The listing builds one solid part. Answer for the finished solid, in the listing's coordinates (mm). A direction names the side the tool comes from. Round coordinates to 2 decimals unless told otherwise and drop trailing zeros. Order: outer loops, then holes, each group sorted by start corner. A loop starts at its lowest first (then second) coordinate and runs counter-clockwise, first axis right, second up. Notation, with made-up numbers: M 28.5,-16 L 36.5,-16 A20 cw 36.5,-3 Z; hole C 46.25,57.5 d4. An arc over 180 degrees is marked long. Put each result on its own line as item: value. Start each with the question number.
1. Each of these flat-tipped pins is pushed along its axis until it touches: pin 1 Ø4 at (x, z) = (1.5, 3) entering from +Y; pin 2 Ø2 at (x, z) = (-1, 3) entering from -Y; pin 3 Ø3 at (x, z) = (2.5, 3) entering from +Y. Where does it stop, or does it pass through?
2. Which of the six approach directions +Z, -Z, +X, -X, +Y, -Y give full straight-line access (tool end or side, diameter ignored) to faces 5 (the face through (2, -2, 6)), 6 (the face through (0, -2, 8.2)), 7 (the face through (0, 0, 6.9))?
3. The part is cut by section A-A (z = 7.75). Give the vertices of the cut face in (x, y), then the cut area to 3 significant figures.
4. The part is cut by section C-C (z = 2.5). Give the vertices of the cut face in (x, y), then the cut area to 3 significant figures.
5. The mould has two halves that part along X. Classify faces 1 (the face through (-1.088, -0.616, 7.541)), 2 (the face through (0, -2, 3)), 3 (the face through (-1.08, 0.63, 7.54)), 4 (the face through (0, 0, 0)): +X half, -X half, draft (parallel to the pull), parting line (faces both ways), or undercut.
6. The part is cut by section B-B (x = 0). Give the vertices of the cut face in (y, z).
7. Consider line 1 (Z direction, x = -0.5, y = -1); line 2 (Y direction, x = 0, z = 5.75); line 3 (X direction, y = -0.5, z = 3.5). Determine where each line is inside the solid, lowest interval first.
from build123d import *

# Parameters (mm, degrees)
SKETCH1_R      = 2
SHANK_DEPTH    = 6
SKETCH2_R      = 3.8
HEAD_DEPTH     = 2.2
BUTTON_ROUND_R = 1.5
SOCKET_DEPTH   = 1.3


with BuildPart() as part:
    # Sketch1 → Shank (new body)
    with BuildSketch(Plane.XY):
        Circle(SKETCH1_R)
    extrude(amount=SHANK_DEPTH)

    # Sketch2 → Head (add)
    with BuildSketch(Plane.XY.offset(6)):
        Circle(SKETCH2_R)
    extrude(amount=HEAD_DEPTH)

    # Button_round
    button_round_edges = [part.edges().sort_by_distance(p)[0] for p in [
        (-3.8, 0, 8.2),
    ]]
    fillet(button_round_edges, radius=BUTTON_ROUND_R)

    # Sketch3 → Socket (cut)
    with BuildSketch(Plane.XY.offset(6.9)):
        Polygon((1.443375673, 0), (0.721687836, 1.25), (-0.721687836, 1.25), (-1.443375673, 0), (-0.721687836, -1.25), (0.721687836, -1.25), align=None)
    extrude(amount=SOCKET_DEPTH, mode=Mode.SUBTRACT)


solid = part.part
Resolved:
1. pin 1: y = 2
1. pin 2: y = -2
1. pin 3: y = 1.73
2. face 5: -Z
2. face 6: +Z, +X, -X, +Y, -Y
2. face 7: +Z
3. outline: C 0,0 d6.74; hole M -1.44,0 L -0.72,-1.25 L 0.72,-1.25 L 1.44,0 L 0.72,1.25 L -0.72,1.25 Z
3. area: 30.3 mm2
4. outline: C 0,0 d4
4. area: 12.6 mm2
5. face 1: undercut
5. face 2: parting line
5. face 3: undercut
5. face 4: draft
6. outline: M -3.8,6 L -2,6 L -2,0 L 2,0 L 2,6 L 3.8,6 L 3.8,6.7 A1.5 ccw 2.3,8.2 L 1.25,8.2 L 1.25,6.9 L -1.25,6.9 L -1.25,8.2 L -2.3,8.2 A1.5 ccw -3.8,6.7 Z
7. line 1: 0 to 6.9
7. line 2: -2 to 2
7. line 3: -1.94 to 1.94
